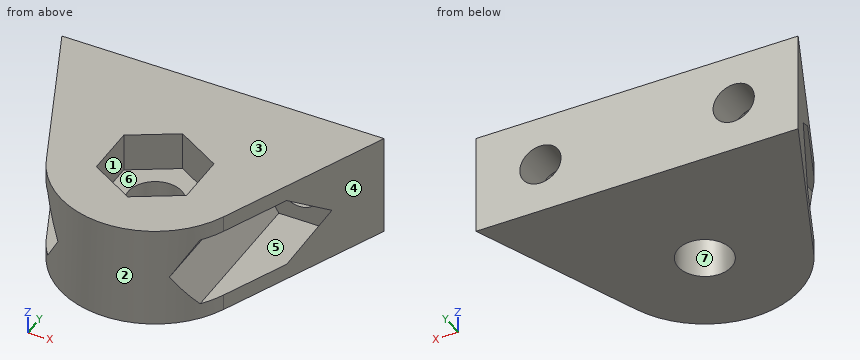
from build123d import *

# Parameters (mm, degrees)
SKETCH1_R           = 2.1
BOSS_EXTRUDE1_DEPTH = 8
SKETCH2_R           = 1.6
CUT_EXTRUDE1_DEPTH  = 18.5
CUT_EXTRUDE2_DEPTH  = 3
CUT_EXTRUDE3_START  = -3
CUT_EXTRUDE3_DEPTH  = 15.5000001


with BuildPart() as part:
    # Sketch1 → Boss-Extrude1 (new body)
    with BuildSketch(Plane.XY):
        with BuildLine():
            Line((-6.883064085, -2.978830106), (-12.5, 10))
            Line((-12.5, 10), (12.5, 10))
            Line((12.5, 10), (6.883064085, -2.978830106))
            ThreePointArc((6.883064085, -2.978830106), (0, -7.5), (-6.883064085, -2.978830106))
        make_face()
        Circle(SKETCH1_R, mode=Mode.SUBTRACT)
    extrude(amount=BOSS_EXTRUDE1_DEPTH)

    # Sketch2 → Cut-Extrude1 (cut, through all)
    with BuildSketch(Plane(origin=(0, 10, 0), x_dir=(1, 0, 0), z_dir=(0, 1, 0))):
        with Locations((-7.5, -4)):
            Circle(SKETCH2_R)
        with Locations((7.5, -4)):
            Circle(SKETCH2_R)
    extrude(amount=-CUT_EXTRUDE1_DEPTH, mode=Mode.SUBTRACT)

    # Sketch3 → Cut-Extrude2 (cut)
    with BuildSketch(Plane.XY.offset(8)):
        Polygon((0, -4.041451884), (3.5, -2.020725942), (3.5, 2.020725942), (0, 4.041451884), (-3.5, 2.020725942), (-3.5, -2.020725942), align=None)
    extrude(amount=-CUT_EXTRUDE2_DEPTH, mode=Mode.SUBTRACT)

    # Sketch4 → Cut-Extrude3 (cut, through all)
    with BuildSketch(Plane(origin=(0, 10, 0), x_dir=(1, 0, 0), z_dir=(0, 1, 0)).offset(CUT_EXTRUDE3_START)):
        Polygon((-5.91228676, -6.75), (-4.324573519, -4), (-5.91228676, -1.25), (-9.08771324, -1.25), (-10.675426481, -4), (-9.08771324, -6.75), align=None)
        Polygon((9.08771324, -6.75), (5.91228676, -6.75), (4.324573519, -4), (5.91228676, -1.25), (9.08771324, -1.25), (10.675426481, -4), align=None)
    extrude(amount=-CUT_EXTRUDE3_DEPTH, mode=Mode.SUBTRACT)


solid = part.part
Read the model definition and answer for the solid it produces. Units are mm, in the model's axes. Face numbers are marked on the shaded views. A direction names the side the tool comes from. Coordinates: 2 decimals unless noted, no trailing zeros. Loops run counter-clockwise (first coordinate to the right, second up) from the corner with the lowest first, then second, coordinate; pieces in that order, holes last.
Q1. Which of the six approach directions +Z, -Z, +X, -X, +Y, -Y give full straight-line access (tool end or side, diameter ignored) to the marked faces 5, 6 and 7?
Q2. The part is cut by section A-A on z = 7.5. Write down the section's boundary in (x, y), and give its area (3 significant figures).
Q3. The part is cut by section C-C on y = 0. Write down the section's boundary in (x, z), and give its area (3 significant figures).
Q4. Each of these flat-tipped pins is pushed along its axis until it touches: pin 1 Ø6.5 at (x, y) = (0, 0) entering from -Z; pin 2 Ø3 at (y, z) = (-1, 2.5) entering from -X; pin 3 Ø2.5 at (y, z) = (1, 6.5) entering from +X; pin 4 Ø2 at (y, z) = (5, 1.5) entering from -X. Where does it stop, or does it pass through?
Q5. The part is cut by section B-B on x = -0.5. Write down the section's boundary in (y, z), and give its area (3 significant figures).
Q6. Consider probe 1 along X at (y, z) = (8.1, 4); probe 2 along Z at (x, y) = (7.5, 9.1); probe 3 along Z at (x, y) = (-8.25, 6.5). Determine where each line is inside the solid, lowest interval first.
Q7. The mould has two halves that part along X. Classify the marked faces 1, 2, 3 and 4: +X half, -X half, draft (parallel to the pull), parting line (faces both ways), or undercut.
Q8. The part is cut by section D-D on x = 10. Write down the section's boundary in (y, z), and give its area (3 significant figures).
Results below:
1. face 5: -Y
1. face 6: +Z
1. face 7: +Z, -Z
2. outline: (-12.5, 10) - (-6.88, -2.98) arc R7.5 ccw to (6.88, -2.98) - (12.5, 10) - close; hole (-3.5, -2.02) - (0, -4.04) - (3.5, -2.02) - (3.5, 2.02) - (0, 4.04) - (-3.5, 2.02) - close
2. area: 254 mm2
3. outline: (-8.17, 0) - (-2.1, 0) - (-2.1, 5) - (-3.5, 5) - (-3.5, 8) - (-8.17, 8) - (-8.17, 6.75) - (-5.91, 6.75) - (-4.32, 4) - (-5.91, 1.25) - (-8.17, 1.25) - close; (2.1, 0) - (8.17, 0) - (8.17, 1.25) - (5.91, 1.25) - (4.32, 4) - (5.91, 6.75) - (8.17, 6.75) - (8.17, 8) - (3.5, 8) - (3.5, 5) - (2.1, 5) - close
3. area: 55.2 mm2
4. pin 1: stops at z = 0
4. pin 2: stops at x = -8.1
4. pin 3: stops at x = 9.14
4. pin 4: stops at x = -10.77
5. outline: (-7.48, 0) - (-2.04, 0) - (-2.04, 5) - (-3.75, 5) - (-3.75, 8) - (-7.48, 8) - close; (2.04, 0) - (10, 0) - (10, 8) - (3.75, 8) - (3.75, 5) - (2.04, 5) - close
5. area: 97.0 mm2
6. probe 1: x = -11.68 to -9.1, -5.9 to 5.9, 9.1 to 11.68
6. probe 2: z = 0 to 2.4, 5.6 to 8
6. probe 3: z = 0 to 1.25, 6.75 to 8
7. face 1: undercut
7. face 2: parting line
7. face 3: draft
7. face 4: +X half
8. outline: (4.22, 0) - (10, 0) - (10, 8) - (4.22, 8) - (4.22, 5.17) - (7, 5.17) - (7, 2.83) - (4.22, 2.83) - close
8. area: 39.7 mm2
